from build123d import *

# Parameters (mm, degrees)
SKETCH1_W           = 14
SKETCH1_H           = 23
BOSS_EXTRUDE1_DEPTH = 14
SKETCH2_W           = 10.4
SKETCH2_H           = 8.65
SKETCH2_W_2         = 8.5
SKETCH2_H_2         = 2.85
CUT_EXTRUDE1_DEPTH  = 20
SKETCH3_W           = 14
SKETCH3_H           = 10.5
SKETCH3_R           = 1.5
BOSS_EXTRUDE2_DEPTH = 2
BOSS_EXTRUDE3_DEPTH = 1.5
SKETCH5_W           = 8.5
SKETCH5_H           = 11.5
CUT_EXTRUDE2_DEPTH  = 4


with BuildPart() as part:
    # Sketch1 → Boss-Extrude1 (new body)
    with BuildSketch(Plane.XY):
        Rectangle(SKETCH1_W, SKETCH1_H)
    extrude(amount=BOSS_EXTRUDE1_DEPTH)

    # Sketch2 → Cut-Extrude1 (cut)
    with BuildSketch(Plane.XZ.offset(11.5)):
        with Locations((0, 7.175)):
            Rectangle(SKETCH2_W, SKETCH2_H)
        with Locations((0, 1.425)):
            Rectangle(SKETCH2_W_2, SKETCH2_H_2)
    extrude(amount=-CUT_EXTRUDE1_DEPTH, mode=Mode.SUBTRACT)

    # Sketch3 → Boss-Extrude2 (add)
    with BuildSketch(Plane.XZ.offset(11.5)):
        with Locations((0, 19.25)):
            Rectangle(SKETCH3_W, SKETCH3_H)
        with Locations((0, 20)):
            Circle(SKETCH3_R, mode=Mode.SUBTRACT)
    extrude(amount=-BOSS_EXTRUDE2_DEPTH)

    # Sketch4 → Boss-Extrude3 (add)
    with BuildSketch(Plane.ZY.offset(7)):
        with BuildLine():
            Line((14, -3.5), (14, -9.5))
            Line((14, -9.5), (20, -9.5))
            ThreePointArc((20, -9.5), (15.757359313, -7.742640687), (14, -3.5))
        make_face()
    boss_extrude3 = extrude(amount=-BOSS_EXTRUDE3_DEPTH)

    # Mirror1: Boss-Extrude3 across plane
    add(boss_extrude3.mirror(Plane(origin=(0, 0, 0), x_dir=(0, 0, 1), z_dir=(1, 0, 0))))

    # Sketch5 → Cut-Extrude2 (cut, through all)
    with BuildSketch(Plane.XZ.offset(-8.5)):
        with Locations((0, 5.75)):
            Rectangle(SKETCH5_W, SKETCH5_H)
    extrude(amount=-CUT_EXTRUDE2_DEPTH, mode=Mode.SUBTRACT)


solid = part.part
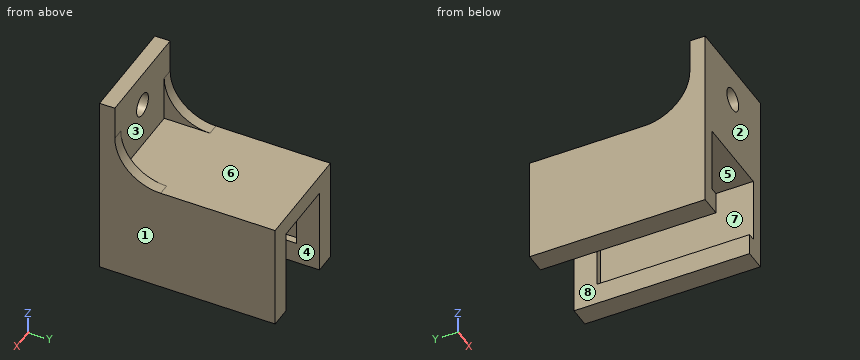
Input: part model. Units: mm. Frame: model coordinates. Face numbers are marked on the shaded views. A direction names the side the tool comes from. Give positions to 0.01 mm unless a question says otherwise; leave off trailing zeros. Loops run counter-clockwise (first coordinate to the right, second up) from the corner with the lowest first, then second, coordinate; pieces in that order, holes last. Notation, with made-up numbers: (36.25, -15) - (50.25, -15) arc R18 ccw to (50.25, -1) - close; hole circle Ø6 at (72, 43). An arc over 180 degrees is marked (long way). Use CSV: the item, a comma, the result in double quotes. Start each with the question number.
Item 1: Contact query for flat-ended pins moving along their axis: P1, Ø7, axis at x = 1, y = 0.5, coming from the +Z side; P2, Ø1, axis at x = 4.5, z = 7, coming from the -Y side; P3, Ø2.5, axis at x = 0, z = 20, coming from the -Y side. Output: stop coordinate, or through.
Item 2: Line query: line 1 (X direction, y = -3.25, z = 5.75); line 2 (Z direction, x = 0, y = -10.7); line 3 (Z direction, x = 3.5, y = 0.25). Output: solid intervals per line, ascending.
Item 3: Section C-C on y = 9.5. Return loops of the section in (x, z).
Item 4: Reachability of the marked faces 1, 2, 3, 4 and 5 from +Z, -Z, +X, -X, +Y, -Y: full face, straight path, thin tool, end or side. Return the list, or none.
Item 5: Section D-D on x = -2.5. Return loops of the section in (y, z).
Item 6: Section B-B on x = 0. Return loops of the section in (y, z), then the cut area to 3 significant figures.
Item 7: Section A-A on z = 5.25. Return loops of the section in (x, y).
Item 8: Mould query, pull axis Z, two halves, no side actions, for the marked faces 6, 7 and 8. Classes: pulls with the +Z half, pulls with the -Z half, needs draft (parallel to the pull), parting line crosses it, or undercut.
Ans:
1,P1,"stops at z = 14"
1,P2,"stops at y = 8.5"
1,P3,"passes through"
2,line 1,"x = -7 to -5.2, 5.2 to 7"
2,line 2,"z = 11.5 to 18.5, 21.5 to 24.5"
2,line 3,"z = 11.5 to 14"
3,outline,"(-7, 0) - (-4.25, 0) - (-4.25, 11.5) - (4.25, 11.5) - (4.25, 0) - (7, 0) - (7, 14) - (-7, 14) - close"
4,face 1,"+Z, -Z, +X, +Y, -Y"
4,face 2,"+Z, -Z, +X, -X, -Y"
4,face 3,"+Z, +Y"
4,face 4,"-Z, +Y, -Y"
4,face 5,"-Y"
5,outline,"(-11.5, 11.5) - (11.5, 11.5) - (11.5, 14) - (-9.5, 14) - (-9.5, 24.5) - (-11.5, 24.5) - close"
6,outline,"(-11.5, 11.5) - (11.5, 11.5) - (11.5, 14) - (-9.5, 14) - (-9.5, 18.5) - (-11.5, 18.5) - close; (-11.5, 21.5) - (-9.5, 21.5) - (-9.5, 24.5) - (-11.5, 24.5) - close"
6,area,"72.5 mm2"
7,outline,"(-7, -11.5) - (-5.2, -11.5) - (-5.2, 8.5) - (-4.25, 8.5) - (-4.25, 11.5) - (-7, 11.5) - close; (4.25, 8.5) - (5.2, 8.5) - (5.2, -11.5) - (7, -11.5) - (7, 11.5) - (4.25, 11.5) - close"
8,face 6,"pulls with the +Z half"
8,face 7,"undercut"
8,face 8,"needs draft"
